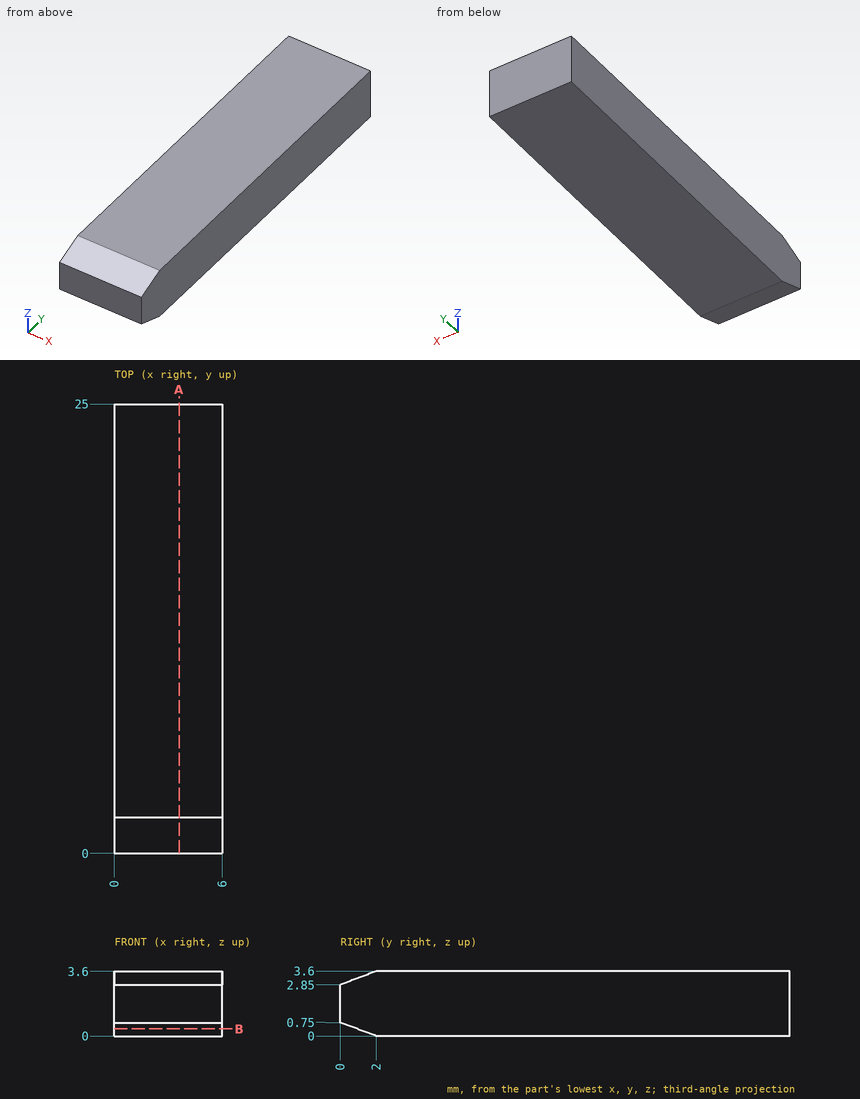
Check sheet for the drawn part. Datum: minimum x, y, z corner. Units: mm. Round coordinates to 2 decimals unless told otherwise and drop trailing zeros. Order: outer loops, then holes, each group sorted by start corner. A loop starts at its lowest first (then second) coordinate and runs counter-clockwise, first axis right, second up. Notation, with made-up numbers: M -2.5,6.5 L 36.5,6.5 A21 cw 36.5,28.5 Z; hole C 33.5,-33 d11. An arc over 180 degrees is marked long. Write each question's results on one line, items separated by ' | '. Start each with the question number.
1. Cross-section at B-B on z = 0.4. Record the boundary of the cut face in (x, y), plus the area to 3 significant figures.
2. Cross-section at A-A on x = 3.6. Record the boundary of the cut face in (y, z), plus the area to 3 significant figures.
3. Go/stop test with a flat-tipped pin: P1, Ø1.5, axis at x = 4, z = 2, coming from the -Y side. Record where the tip stops, or that it passes through.
Resolved:
1) outline: M 0,0.93 L 6,0.93 L 6,25 L 0,25 Z | area: 144 mm2
2) outline: M 0,0.75 L 2,0 L 25,0 L 25,3.6 L 2,3.6 L 0,2.85 Z | area: 88.5 mm2
3) P1: y = 0
